Geometry check sheet. Reference: drawing and pictorial views, mm from the part's lowest x, y, z. A direction names the side the tool comes from. Give positions to 0.01 mm unless a question says otherwise; leave off trailing zeros. Order: outer loops, then holes, each group sorted by start corner. A loop starts at its lowest first (then second) coordinate and runs counter-clockwise, first axis right, second up.
Item 1: Material ranges on line 1 along Z through (x, y) = (8, 20.75); line 2 along Y through (x, z) = (10, 24.25); line 3 along Y through (x, z) = (3.75, 2), recorded low to high.
Item 2: Access from +Z, -Z, +X, -X, +Y, -Y to the whole of each face (thin tool, end or side, straight path). Record for the marked faces 1, 2 and 3.
Item 3: Gauge pin test, flat ends, axial feed: P1, Ø7.5, axis at x = 10, y = 17.47, coming from the -Z side; P2, Ø4, axis at x = 10, z = 21, coming from the +Y side; P3, Ø3, axis at x = 16, y = 10.5, coming from the +Z side. Record the tip position at first contact, or that the pin passes through.
Item 4: Sectioned sample at B-B on y = 3. Record the boundary of the cut face in (x, z), and give its area (3 significant figures).
Item 5: Sectioned sample at C-C on z = 25. Record the boundary of the cut face in (x, y).
Item 6: Release check for a two-part mould opening along Z. For the marked faces 4, 5 and 6 record: released by +Z, released by -Z, zero draft, split by the parting line, or undercut.
Item 7: Sectioned sample at A-A on x = 10. Record the boundary of the cut face in (y, z), and give its area (3 significant figures).
Item 8: Sectioned sample at D-D on x = 4.75. Record the boundary of the cut face in (y, z).
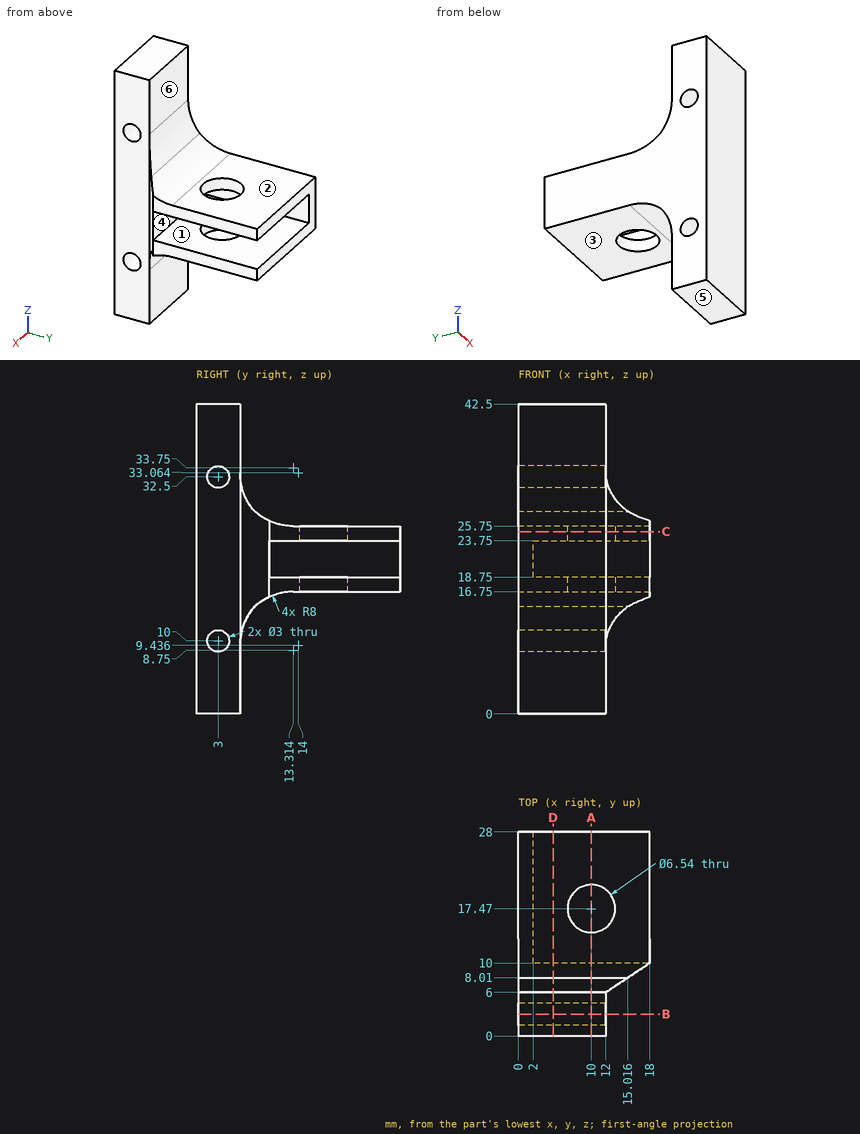
Report:
1. line 1: z = 16.75 to 18.75, 23.75 to 25.75
1. line 2: y = 0 to 14.2, 20.74 to 28
1. line 3: y = 0 to 6
2. face 1: +X, +Y
2. face 2: +Z, +X, -X, +Y
2. face 3: -Z, +X, -X, +Y
3. P1: stops at z = 16.75
3. P2: stops at y = 10
3. P3: stops at z = 27.01
4. outline: (0, 0) - (12, 0) - (12, 8.5) - (0, 8.5) - close; (0, 11.5) - (12, 11.5) - (12, 31) - (0, 31) - close; (0, 34) - (12, 34) - (12, 42.5) - (0, 42.5) - close
4. area: 438 mm2
5. outline: (0, 0) - (12, 0) - (12, 6) - (18, 10) - (18, 28) - (0, 28) - close; hole circle Ø6.54 at (10, 17.47)
6. face 4: undercut
6. face 5: released by -Z
6. face 6: zero draft
7. outline: (0, 0) - (6, 0) - (6, 9.44) arc R8 cw to (8.01, 14.74) arc R8 cw to (13.31, 16.75) - (14.2, 16.75) - (14.2, 18.75) - (10, 18.75) - (10, 23.75) - (14.2, 23.75) - (14.2, 25.75) - (13.31, 25.75) arc R8 cw to (8.01, 27.76) arc R8 cw to (6, 33.06) - (6, 42.5) - (0, 42.5) - close; (20.74, 16.75) - (28, 16.75) - (28, 18.75) - (20.74, 18.75) - close; (20.74, 23.75) - (28, 23.75) - (28, 25.75) - (20.74, 25.75) - close; hole circle Ø3 at (3, 10); hole circle Ø3 at (3, 32.5)
7. area: 344 mm2
8. outline: (0, 0) - (6, 0) - (6, 9.44) arc R8 cw to (8.01, 14.74) arc R8 cw to (13.31, 16.75) - (28, 16.75) - (28, 18.75) - (10, 18.75) - (10, 23.75) - (28, 23.75) - (28, 25.75) - (13.31, 25.75) arc R8 cw to (8.01, 27.76) arc R8 cw to (6, 33.06) - (6, 42.5) - (0, 42.5) - close; hole circle Ø3 at (3, 10); hole circle Ø3 at (3, 32.5)
